from build123d import *

# Parameters (mm, degrees)
SKETCH_1_W          = 50
SKETCH_1_H          = 150
EXTRUDE_1_DEPTH     = 5
SKETCH_2_R          = 3.75
CUT_EXTRUDE_1_DEPTH = 5
SKETCH_3_R          = 4
CUT_EXTRUDE_2_DEPTH = 5
SKETCH_4_W          = 15
SKETCH_4_H          = 6
CUT_EXTRUDE_3_DEPTH = 5
SKETCH_5_R          = 5.24
CUT_EXTRUDE_4_DEPTH = 5


with BuildPart() as part:
    # 草图1 → 凸台-拉伸1 (new body)
    with BuildSketch(Plane.XY):
        with Locations((1.67844523, -33.188535046)):
            Rectangle(SKETCH_1_W, SKETCH_1_H)
    extrude(amount=EXTRUDE_1_DEPTH)

    # 草图2 → 切除-拉伸1 (cut)
    with BuildSketch(Plane.XY.offset(5)):
        with Locations((-13.32155477, -93.188535046)):
            Circle(SKETCH_2_R)
        with Locations((-13.32155477, -80.188535046)):
            Circle(SKETCH_2_R)
        with Locations((-13.32155477, -68.648535046)):
            Circle(SKETCH_2_R)
        with Locations((-13.32155477, 2.849464954)):
            Circle(SKETCH_2_R)
        with Locations((-13.32155477, 14.863464954)):
            Circle(SKETCH_2_R)
    extrude(amount=-CUT_EXTRUDE_1_DEPTH, mode=Mode.SUBTRACT)

    # 草图3 → 切除-拉伸2 (cut)
    with BuildSketch(Plane.XY.offset(5)):
        with Locations((-16.82155477, -56.429938563)):
            Circle(SKETCH_3_R)
        with Locations((-16.82155477, -33.139938563)):
            Circle(SKETCH_3_R)
    extrude(amount=-CUT_EXTRUDE_2_DEPTH, mode=Mode.SUBTRACT)

    # 草图4 → 切除-拉伸3 (cut)
    with BuildSketch(Plane.XY.offset(5)):
        with Locations((-13.32155477, -45.429938563)):
            Rectangle(SKETCH_4_W, SKETCH_4_H)
    extrude(amount=-CUT_EXTRUDE_3_DEPTH, mode=Mode.SUBTRACT)

    # 草图5 → 切除-拉伸4 (cut)
    with BuildSketch(Plane.XY.offset(5)):
        with Locations((9.295497906, -12.060281788)):
            Circle(SKETCH_5_R)
        with Locations((9.295497906, -62.477916171)):
            Circle(SKETCH_5_R)
    extrude(amount=-CUT_EXTRUDE_4_DEPTH, mode=Mode.SUBTRACT)


solid = part.part
Build history of the part. All positions in model axes, mm. A direction names the side the tool comes from. Give positions to 0.01 mm unless a question says otherwise; leave off trailing zeros. Write each loop counter-clockwise with the first axis right and the second up, starting at its lowest first coordinate (ties: lowest second). Pieces come first, ordered by that corner, then holes. Notation, with made-up numbers: (77, -16) - (84, -16) arc R5 cw to (84, -12) - close; hole circle Ø9 at (-10, -20). An arc over 180 degrees is marked (long way). Use one line per item in the form item = value. Start each with the question number.
1. Band-saw the part on C-C on z = 3.5. Count the separate pieces of the cut face and the enclosed holes in it, plus the area to 3 significant figures.
2. Two-plate mould, pull along X, no slides. Class faces 3 (the face through (-23.322, -34, 2)), 4 (the face through (26.678, -34, 2)), 5 (the face through (-5.822, -45, 3)), 6 (the face through (1, 41.811, 2)): released by +X, released by -X, zero draft, split by the parting line, or undercut.
3. Band-saw the part on A-A on y = -47. Write the cut outline in (x, z).
4. 3-axis set-ups, long thin cutter, end or side, ignore diameter. For faces 1 (the face through (1, -108.189, 2)), 2 (the face through (-20.822, -45, 3)): which of +Z, -Z, +X, -X, +Y, -Y reach the whole face in a straight line?
5. Band-saw the part on D-D on x = 13. Write the cut outline in (y, z).
6. Band-saw the part on B-B on x = 5.5. Write the cut outline in (y, z), plus the area to 3 significant figures.
7. Probe line 1 (Y direction, x = 7.5, z = 4.8); line 2 (Y direction, x = -19, z = 4.55); line 3 (Y direction, x = 11.5, z = 3.7). List the from-to ranges inside material, lowest first. Write a range as [from, to].
Conclusion:
q1.separate_pieces = 1
q1.enclosed_holes = 10
q1.area = 6,920 mm²
q2.face_3 = released by -X
q2.face_4 = released by +X
q2.face_5 = undercut
q2.face_6 = zero draft
q3.outline = (-23.32, 0) - (-20.82, 0) - (-20.82, 5) - (-23.32, 5) - close; (-5.82, 0) - (26.68, 0) - (26.68, 5) - (-5.82, 5) - close
q4.face_1 = +Z, -Z, +X, -X, -Y
q4.face_2 = +Z, -Z
q5.outline = (-108.19, 0) - (-66.18, 0) - (-66.18, 5) - (-108.19, 5) - close; (-58.77, 0) - (-15.77, 0) - (-15.77, 5) - (-58.77, 5) - close; (-8.35, 0) - (41.81, 0) - (41.81, 5) - (-8.35, 5) - close
q6.outline = (-108.19, 0) - (-66.09, 0) - (-66.09, 5) - (-108.19, 5) - close; (-58.87, 0) - (-15.67, 0) - (-15.67, 5) - (-58.87, 5) - close; (-8.45, 0) - (41.81, 0) - (41.81, 5) - (-8.45, 5) - close
q6.area = 678 mm²
q7.line_1 = [-108.19, -67.4], [-57.56, -16.98], [-7.14, 41.81]
q7.line_2 = [-108.19, -59.78], [-53.08, -48.43], [-42.43, -36.49], [-29.79, 41.81]
q7.line_3 = [-108.19, -67.23], [-57.72, -16.81], [-7.31, 41.81]
